The model under review builds one solid part; all positions refer to its coordinate system, in mm. Give positions to 0.01 mm unless a question says otherwise; leave off trailing zeros. Order: outer loops, then holes, each group sorted by start corner. A loop starts at its lowest first (then second) coordinate and runs counter-clockwise, first axis right, second up. Notation, with made-up numbers: M 38,40 L 92,40 A12 ccw 92,62 Z; hole C -36,68 d7. An arc over 180 degrees is marked long. One line per question, with ' | ' between items. Start each with the question number.
1. The part is to be moulded in two halves that separate along X. For faces 1 (the face through (15, 20, 10)), 2 (the face through (3.01, 10.14, 2.85)), 3 (the face through (33, 10, 10)), say which applies: +X half, -X half, draft (parallel to the pull), parting line (faces both ways), or undercut.
2. We need section D-D on x = 3.5. Write out the cut boundary in (y, z), then the cut area to 3 significant figures.
3. Wall thickness on L1, parallel to Z at x = 10, y = 6; L2, parallel to Y at x = 31, z = 13.75; L3, parallel to Z at x = 8, y = 3: over which ranges is each line inside the solid? List them lowest first.
4. We need section C-C on x = 9. Write out the cut boundary in (y, z).
```python
from build123d import *

# Parameters (mm, degrees)
F0_W     = 39.9999970493
F0_H     = 20
F1_DEPTH = 20
F3_D     = 6
F5_D     = 6
F6_R     = 9.99999
F7_R     = 9.99999


# Not quite as in the source:
# - a fillet or chamfer is up to 0.001 mm smaller than in the source, because OpenCascade refuses the exact size


with BuildPart() as f1:
    # F0 (on Top) → F1 (new body)
    with BuildSketch(Plane.XY):
        with Locations((19.9999985246, 10)):
            Rectangle(F0_W, F0_H)
    extrude(amount=F1_DEPTH)

    # F3 (through all)
    with Locations(Plane.XY.offset(20)):
        with Locations((30.0000011921, 10)):
            Hole(F3_D / 2)

    # F5 (through all)
    with Locations(Plane.XZ):
        with Locations((10, 10)):
            Hole(F5_D / 2)

    # F6 (radius 10 in the source; OpenCascade refuses exactly that, so slightly less here)
    f6_edges = [f1.edges().sort_by_distance(p)[0] for p in [
        (39.999997, 0, 10),
        (39.999997, 20, 10),
    ]]
    fillet(f6_edges, radius=F6_R)

    # F7 (radius 10 in the source; OpenCascade refuses exactly that, so slightly less here)
    f7_edges = [f1.edges().sort_by_distance(p)[0] for p in [
        (0, 10, 0),
        (0, 10, 20),
    ]]
    fillet(f7_edges, radius=F7_R)


solid = f1.part
```
Entries:
1) face 1: draft | face 2: -X half | face 3: undercut
2) outline: M 0,2.4 L 20,2.4 L 20,17.6 L 0,17.6 Z | area: 304 mm^2
3) L1: z = 0 to 7, 13 to 20 | L2: y = 0.05 to 7.17, 12.83 to 19.95 | L3: z = 0.2 to 7.76, 12.24 to 19.8
4) outline: M 0,0.05 L 20,0.05 L 20,7.17 L 0,7.17 Z; M 0,12.83 L 20,12.83 L 20,19.95 L 0,19.95 Z
